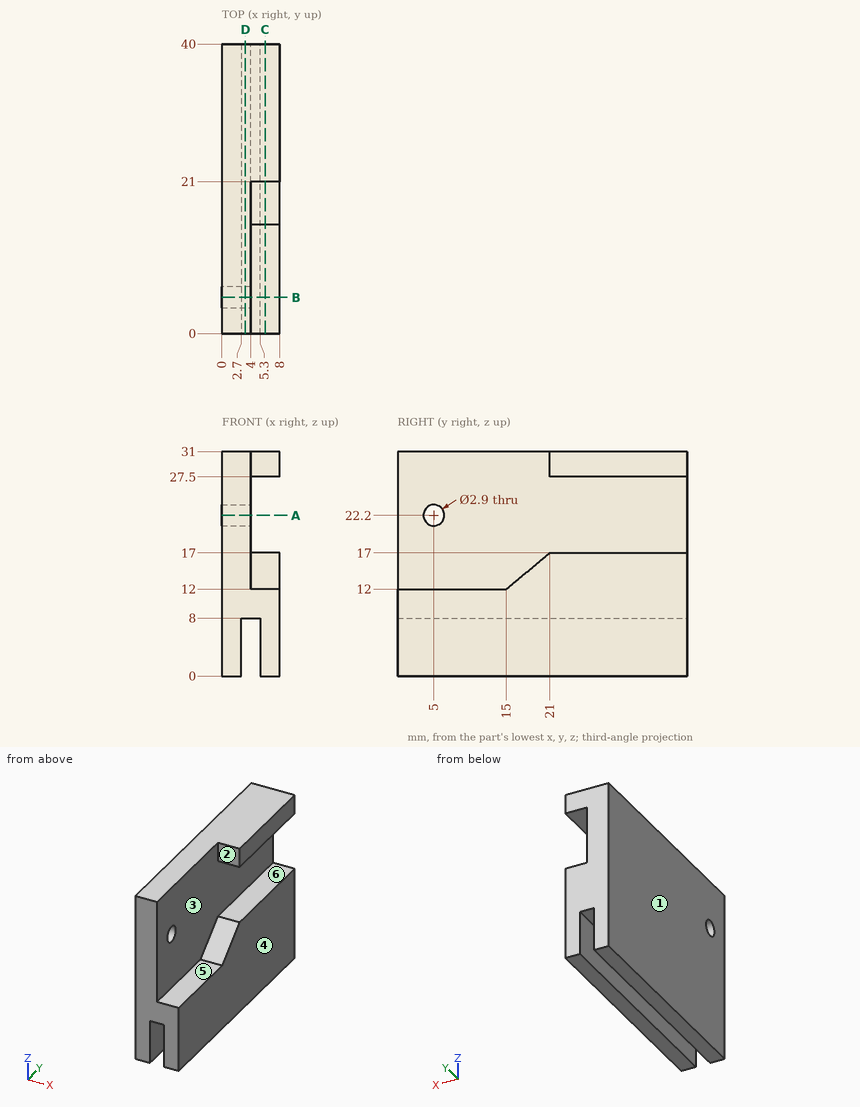
Study the drawing (mm; zero at the part's minimum x, y, z) and answer. A direction names the side the tool comes from. Give positions to 0.01 mm unless a question says otherwise; leave off trailing zeros. Loops run counter-clockwise (first coordinate to the right, second up) from the corner with the lowest first, then second, coordinate; pieces in that order, holes last. Notation, with made-up numbers: (48.25, -23.5) - (56.25, -23.5) arc R20 cw to (56.25, 3.5) - close; hole circle Ø5 at (58, -25.75). An arc over 180 degrees is marked (long way). Return JSON: item names as keys, results as strings. Group by question number.
1. Given pin 1 Ø0.8 at (x, y) = (4.5, 17.5) entering from -Z; pin 2 Ø4 at (x, z) = (7, 29) entering from -Y; pin 3 Ø1.5 at (x, y) = (5, 5) entering from +Z, each flat-ended and moving along its own axis, determine where each tip first touches the part or whether it passes through.
2. Determine the mould class of the marked faces 3, 4, 5 and 6 for opening direction Z: pulls with the +Z half, pulls with the -Z half, needs draft (parallel to the pull), parting line crosses it, or undercut.
3. Find section A-A (z = 22.2). Write down the section's boundary in (x, y).
4. Find section C-C (x = 6). Write down the section's boundary in (y, z).
5. Straight lines are drawn through the part: line 1 (X direction, y = 37, z = 5); line 2 (Z direction, x = 2.2, y = 5); line 3 (Z direction, x = 4.75, y = 31.5). For each, find the intervals that lie inside material, in ascending order. Write a range as [from, to].
6. Find section B-B (y = 5). Write down the section's boundary in (x, z), then the cut area to 3 significant figures.
7. Find section D-D (x = 3.25). Write down the section's boundary in (y, z).
8. Which of the six approach directions +Z, -Z, +X, -X, +Y, -Y give full straight-line access (tool end or side, diameter ignored) to the marked faces 1 and 2?
Verdict:
{
 "1": {"pin 1": "stops at z = 8", "pin 2": "stops at y = 21", "pin 3": "stops at z = 12"},
 "2": {"face 3": "undercut", "face 4": "needs draft", "face 5": "pulls with the +Z half", "face 6": "undercut"},
 "3": {"outline": "(0, 0) - (4, 0) - (4, 3.55) - (0, 3.55) - close; (0, 6.45) - (4, 6.45) - (4, 40) - (0, 40) - close"},
 "4": {"outline": "(0, 0) - (40, 0) - (40, 17) - (21, 17) - (15, 12) - (0, 12) - close; (21, 27.5) - (40, 27.5) - (40, 31) - (21, 31) - close"},
 "5": {"line 1": "x = [0, 2.7], [5.3, 8]", "line 2": "z = [0, 20.75], [23.65, 31]", "line 3": "z = [8, 17], [27.5, 31]"},
 "6": {"outline": "(0, 0) - (2.7, 0) - (2.7, 8) - (5.3, 8) - (5.3, 0) - (8, 0) - (8, 12) - (4, 12) - (4, 20.75) - (0, 20.75) - close; (0, 23.65) - (4, 23.65) - (4, 31) - (0, 31) - close", "area": "140 mm^2"},
 "7": {"outline": "(0, 8) - (40, 8) - (40, 31) - (0, 31) - close; hole circle Ø2.9 at (5, 22.2)"},
 "8": {"face 1": "+Z, -Z, -X, +Y, -Y", "face 2": "+Z, +X, -Y"}
}
